For this review, take the finished solid that the model builds, in its own axes (mm). A direction names the side the tool comes from. Round coordinates to 2 decimals unless told otherwise and drop trailing zeros. Loops run counter-clockwise (first coordinate to the right, second up) from the corner with the lowest first, then second, coordinate; pieces in that order, holes last.
1) Mouldability with a two-part tool opening along X and no side actions: class faces 1 (the flat face through (10, -107, 198)), 2 (the flat face through (0, -107, 107.112)), 3 (the flat face through (134.18, -58.76, 182.79)), 4 (the flat face through (1, -107, 237.112)) as pulls with the +X half, pulls with the -X half, needs draft (parallel to the pull), parting line crosses it, or undercut.
2) Take a section at B-B (z = 196). State the section outline as (x, y) points, then the cut area to 3 significant figures.
3) Tool access review of faces 5 (the flat face through (59.507, -155.203, 101.899)), 6 (the flat face through (-200.001, -106.981, -24.255)), 7 (the flat face through (-40, -107, 217.112)): name each direction out of +Z, -Z, +X, -X, +Y, -Y from which nothing blocks a thin tool from reaching the whole face with its end or side.
4) Wall thickness on L1, parallel to X at y = -101, z = 132.5; L2, parallel to X at y = -12.5, z = 139; L3, parallel to X at y = -186, z = 171: over which ranges is each line inside the solid? List them lowest first.
5) Take a section at C-C (x = 141). Give the number of separate pieces and of enclosed holes in the cut face, then the cut area to 3 significant figures.
6) Insertion check: pin 1 (12 mm diameter, centred on x = -164, y = -76.5, fed in from +Z); pin 2 (6 mm diameter, centred on x = -3, y = -85.5, fed in from -Z); pin 3 (4 mm diameter, centred on x = 107.5, y = -49, fed in from +Z). Each pin has a flat end and moves straight along its axis. Give the tip position at first contact, or say it passes through.
7) Take a section at A-A (y = -201). State the section outline as (x, z) points.
```python
from build123d import *

# Parameters (mm, degrees)
F1_DEPTH = 217
F2_R     = 85
F3_DEPTH = 120
F4_R     = 85
F5_DEPTH = 120


with BuildPart() as f1:
    # F0 (on Front) → F1 (new body)
    with BuildSketch(Plane.XZ):
        with BuildLine():
            Line((-79.857185, 237.112019), (-270.612759, 46.356446))
            Line((-270.612759, 46.356446), (-256.470623, 32.21431))
            Line((-256.470623, 32.21431), (-73.03738, 215.647553))
            ThreePointArc((-73.03738, 215.647553), (-71.415263, 216.731417), (-69.501846, 217.112019))
            Line((-69.501846, 217.112019), (-10, 217.112019))
            Line((-10, 217.112019), (-10, 179.689983))
            Line((-10, 179.689983), (-23.539905, 166.150078))
            Line((-23.539905, 166.150078), (-206.973149, -17.283164))
            Line((-206.973149, -17.283164), (-192.831013, -31.4253))
            Line((-192.831013, -31.4253), (-10, 151.405712))
            Line((-10, 151.405712), (-10, 107.112019))
            Line((-10, 107.112019), (0, 107.112019))
            Line((0, 107.112019), (10, 107.112019))
            Line((10, 107.112019), (10, 151.405712))
            Line((10, 151.405712), (192.831013, -31.4253))
            Line((192.831013, -31.4253), (206.973149, -17.283164))
            Line((206.973149, -17.283164), (23.539905, 166.150078))
            Line((23.539905, 166.150078), (10, 179.689983))
            Line((10, 179.689983), (10, 217.112019))
            Line((10, 217.112019), (69.501846, 217.112019))
            ThreePointArc((69.501846, 217.112019), (71.415263, 216.731417), (73.03738, 215.647553))
            Line((73.03738, 215.647553), (256.470622, 32.21431))
            Line((256.470622, 32.21431), (270.612758, 46.356446))
            Line((270.612758, 46.356446), (79.857185, 237.112019))
            Line((79.857185, 237.112019), (-79.857185, 237.112019))
        make_face()
    extrude(amount=F1_DEPTH)

    # F2 (on face) → F3 (cut)
    with BuildSketch(Plane(origin=(-158.484602, 0, 158.484603), x_dir=(0.707107, 0, 0.707107), z_dir=(-0.707107, 0, 0.707107))):
        with Locations((-45.80316, -108.5)):
            Circle(F2_R)
    extrude(amount=-F3_DEPTH, mode=Mode.SUBTRACT)

    # F4 (on face) → F5 (cut)
    with BuildSketch(Plane(origin=(158.484602, 0, 158.484602), x_dir=(0.707107, 0, -0.707107), z_dir=(0.707107, 0, 0.707107))):
        with Locations((45.803159, -108.5)):
            Circle(F4_R)
    extrude(amount=-F5_DEPTH, mode=Mode.SUBTRACT)


solid = f1.part
```
Response:
1. face 1: undercut
1. face 2: undercut
1. face 3: pulls with the +X half
1. face 4: needs draft
2. outline: (-120.97, -217) - (-92.68, -217) - (-92.68, 0) - (-120.97, 0) - close; (-10, -217) - (10, -217) - (10, 0) - (-10, 0) - close; (92.68, -217) - (120.97, -217) - (120.97, 0) - (92.68, 0) - close
2. area: 16,600 mm2
3. face 5: -Z, +Y, -Y
3. face 6: -Z, -X, +Y, -Y
3. face 7: +Y, -Y
4. L1: x = -57.19 to -28.91, -10 to 10, 28.91 to 57.19
4. L2: x = -177.97 to -149.68, -50.69 to -22.41, -10 to 10, 22.41 to 50.69, 149.68 to 177.97
4. L3: x = -145.97 to -117.68, -18.69 to 18.69, 117.68 to 145.97
5. separate pieces: 4
5. enclosed holes: 0
5. area: 4,440 mm2
6. pin 1: stops at z = -5.12
6. pin 2: stops at z = 107.11
6. pin 3: stops at z = 211.47
7. outline: (-270.61, 46.36) - (-256.47, 32.21) - (-73.04, 215.65) arc R5 cw to (-69.5, 217.11) - (-10, 217.11) - (-10, 179.69) - (-206.97, -17.28) - (-192.83, -31.43) - (-10, 151.41) - (-10, 107.11) - (10, 107.11) - (10, 151.41) - (192.83, -31.43) - (206.97, -17.28) - (10, 179.69) - (10, 217.11) - (69.5, 217.11) arc R5 cw to (73.04, 215.65) - (256.47, 32.21) - (270.61, 46.36) - (79.86, 237.11) - (-79.86, 237.11) - close
